Can you work these out from the model? Positions are in its coordinate system, mm. A direction names the side the tool comes from. Round coordinates to 2 decimals unless told otherwise and drop trailing zeros. Write each loop counter-clockwise with the first axis right and the second up, starting at its lowest first coordinate (ties: lowest second). Pieces come first, ordered by that corner, then holes. Notation, with made-up numbers: M 46.5,41 L 77.5,41 A7 cw 77.5,52 Z; hole C -14,54.5 d6. An arc over 180 degrees is marked long. Answer in a Markdown table with one row per item. Add a question column.
(1) Suppose I cut it at B-B, the plane y = 37. Write out the boundary of the cut face in (x, z).
(2) I'm going to push flat-ended pins straight in: pin 1 (12 mm diameter, centred on y = 33, z = 42.5, fed in from +X); pin 2 (5 mm diameter, centred on y = 24.5, z = 48.5, fed in from +X); pin 3 (10.5 mm diameter, centred on x = 13, y = 22.5, fed in from +Z). Where does each tip first touch, or does it pass through?
(3) Suppose I cut it at C-C, the plane x = 82. Write out the boundary of the cut face in (y, z).
(4) If I drill on probe 1 along Y at (x, z) = (86, 50); probe 2 along Y at (x, z) = (52, 25); probe 3 along X at (y, z) = (8.5, 20), over which ranges is the centre line in solid material (lowest first)?
(5) Suppose I cut it at A-A, the plane z = 91. Write out the boundary of the cut face in (x, y), then the cut area to 3 significant figures.
(6) If we mould it in two halves opening along Z, with no side actions, what happens to faces 5 (the face through (35, 10, 30)), 6 (the face through (41, 36, 15)), 7 (the face through (71, 25, 60))? For each: released by +Z, released by -Z, zero draft, split by the parting line, or undercut.
(7) For faces 1 (the face through (7.4, 32.33, 79.72)), 2 (the face through (52, 20, 51)), 3 (the face through (42.395, 32.832, 58.095)), 4 (the face through (71, 25, 30)), which set-ups out of +Z, -Z, +X, -X, +Y, -Y let a thin tool reach every point of the face, with its end or its side?
(8) Suppose I cut it at D-D, the plane z = 50. Write out the boundary of the cut face in (x, y).
from build123d import *

# Parameters (mm, degrees)
F0_W      = 100
F0_H      = 45
F1_DEPTH  = 100
F2_W      = 65
F2_H      = 20
F3_DEPTH  = 100.001
F4_W      = 35
F4_H      = 40
F5_DEPTH  = 45.001
F7_DEPTH  = 40
F9_DEPTH  = 85
F10_W     = 33
F10_H     = 10
F11_DEPTH = 70
F12_W     = 33
F12_H     = 40
F13_DEPTH = 10
F15_DEPTH = 100.001


with BuildPart() as f1:
    # F0 (on Top) → F1 (new body)
    with BuildSketch(Plane.XY):
        with Locations((50, 22.5)):
            Rectangle(F0_W, F0_H)
    extrude(amount=F1_DEPTH)

    # F2 (on face) → F3 (cut, through all)
    with BuildSketch(Plane.XY.offset(100)):
        with Locations((67.5, 10)):
            Rectangle(F2_W, F2_H)
    extrude(amount=-F3_DEPTH, mode=Mode.SUBTRACT)

    # F4 (on face) → F5 (cut, through all)
    with BuildSketch(Plane.XZ):
        with Locations((17.5, 80)):
            Rectangle(F4_W, F4_H)
    extrude(amount=-F5_DEPTH, mode=Mode.SUBTRACT)

    # F6 (on face) → F7 (join)
    with BuildSketch(Plane.XY.offset(60)):
        Polygon((0, 20), (15, 45), (0, 45), align=None)
    extrude(amount=F7_DEPTH)

    # F8 (on face) → F9 (cut)
    with BuildSketch(Plane.XY.offset(100)):
        Polygon((35, 21), (50, 45), (35, 45), align=None)
    extrude(amount=-F9_DEPTH, mode=Mode.SUBTRACT)

    # F10 (on face) → F11 (cut)
    with BuildSketch(Plane.XY.offset(100)):
        with Locations((71.5, 25)):
            Rectangle(F10_W, F10_H)
    extrude(amount=-F11_DEPTH, mode=Mode.SUBTRACT)

    # F12 (on face) → F13 (join)
    with BuildSketch(Plane.XZ.offset(-30)):
        with Locations((71.5, 80)):
            Rectangle(F12_W, F12_H)
    extrude(amount=F13_DEPTH)

    # F14 (on face) → F15 (cut, through all)
    with BuildSketch(Plane.XY.offset(100)):
        Polygon((100, 20), (100, 45), (80, 20), align=None)
    extrude(amount=-F15_DEPTH, mode=Mode.SUBTRACT)


solid = f1.part
Calculated:
| question | item | result |
|---|---|---|
| 1 | outline | M 0,0 L 93.6,0 L 93.6,100 L 45,100 L 45,15 L 35,15 L 35,60 L 10.2,60 L 10.2,100 L 0,100 Z |
| 2 | pin 1 | x = 95.2 |
| 2 | pin 2 | x = 55 |
| 2 | pin 3 | z = 60 |
| 3 | outline | M 22.5,0 L 45,0 L 45,100 L 22.5,100 L 22.5,60 L 30,60 L 30,30 L 22.5,30 Z |
| 4 | probe 1 | 30 to 45 |
| 4 | probe 2 | 20 to 45 |
| 4 | probe 3 | 0 to 35 |
| 5 | outline | M 0,20 L 15,45 L 0,45 Z; M 35,20 L 80,20 L 100,45 L 50,45 L 35,21 Z |
| 5 | area | 1,380 mm² |
| 6 | face 5 | zero draft |
| 6 | face 6 | released by +Z |
| 6 | face 7 | undercut |
| 7 | face 1 | +Z, -Y |
| 7 | face 2 | +Z, -Z, +X, -Y |
| 7 | face 3 | +Z, +Y |
| 7 | face 4 | +X, -Y |
| 8 | outline | M 0,0 L 35,0 L 35,20 L 55,20 L 55,30 L 88,30 L 100,45 L 50,45 L 35,21 L 35,45 L 0,45 Z |
